from build123d import *

# Parameters (mm, degrees)
BASE_EXTRUDE_DEPTH = 10.5
FILLET1_R          = 1
SHELL1_START       = 43.20219293
SHELL1_OUTLINE_W   = 8
SHELL1_OUTLINE_H   = 19
SHELL1_DEPTH       = 9


# Read off the part's stored shape, not the designer's step: Shell1
with BuildPart() as part:
    # Sketch1 → Base-Extrude (new, symmetric)
    with BuildSketch(Plane.XY):
        Polygon((17.372143532, -52.78377934), (11.062802732, -43.773106853), (17.616019086, -39.184495362), (23.925359886, -48.195167849), align=None)
    extrude(amount=BASE_EXTRUDE_DEPTH, both=True)

    # Fillet1
    fillet1_edges = [part.edges().sort_by_distance(p)[0] for p in [
        (20.648751709, -50.489473594, 10.5),
        (20.770689486, -43.689831605, 10.5),
        (14.339410909, -41.478801107, 10.5),
        (20.770689486, -43.689831605, -10.5),
        (20.648751709, -50.489473594, -10.5),
        (14.217473132, -48.278443096, -10.5),
        (14.339410909, -41.478801107, -10.5),
        (14.217473132, -48.278443096, 10.5),
        (17.616019086, -39.184495362, 0),
        (23.925359886, -48.195167849, 0),
        (17.372143532, -52.78377934, 0),
        (11.062802732, -43.773106853, 0),
    ]]
    fillet(fillet1_edges, radius=FILLET1_R)

    # Shell1 outline → Shell1 (cut)
    with BuildSketch(Plane(origin=(0, 0, 0), x_dir=(0.8191520442889926, 0.5735764363510448, 0), z_dir=(0.5735764363510448, -0.8191520442889927, 0)).offset(SHELL1_START)):
        with Locations((-12.045105163, 0)):
            Rectangle(SHELL1_OUTLINE_W, SHELL1_OUTLINE_H)
    extrude(amount=SHELL1_DEPTH, mode=Mode.SUBTRACT)


solid = part.part
Verification items for the finished model (mm, model axes). A direction names the side the tool comes from. Round coordinates to 2 decimals unless told otherwise and drop trailing zeros. Loops run counter-clockwise (first coordinate to the right, second up) from the corner with the lowest first, then second, coordinate; pieces in that order, holes last. Notation, with made-up numbers: (17.5, 70) - (64.5, 70) arc R20 ccw to (64.5, 88) - close; hole circle Ø2 at (73.25, 53). An arc over 180 degrees is marked (long way). Write item = value, one per line.
Q1. Depth check by flat-ended pin: pin 1 (4 mm diameter, centred on y = -41, z = -0.5, fed in from -X); pin 2 (4 mm diameter, centred on x = 14.5, z = 3.5, fed in from +Y). Enter the tip coordinate at first touch or a pass-through.
Here are the results:
pin_1 = 12.17
pin_2 = -39.97
Q2. Material ranges on L1, parallel to Z at x = 20.5, y = -45; L2, parallel to Y at x = 17.25, z = 6.75; L3, parallel to Y at x = 17, z = 3.5, recorded low to high.
Here are the results:
L1 = -10.5 to -9.5, 9.5 to 10.5
L2 = -52.32 to -51.65, -40.66 to -39.58
L3 = -52.18 to -51.82, -40.84 to -39.65
Q3. Sectioned sample at A-A on z = -1.25. Record the boundary of the cut face in (x, y).
Here are the results:
outline = (11.64, -44.59) - (18.19, -40) arc R1 ccw to (16.8, -39.76) - (11.88, -43.2) arc R1 ccw to start; (16.8, -51.96) arc R1 ccw to (18.19, -52.21) - (23.11, -48.77) arc R1 ccw to (23.35, -47.38) - close
Q4. Tool access check on faces 1 (the cylindrical face through (20.56, -43.914, 10.215)), 2 (the flat face through (17, -46, 9.5)). Record the directions out of +Z, -Z, +X, -X, +Y, -Y that give a thin tool (end or side, any length) a straight path to the whole face; none if there is none.
Here are the results:
face_1 = +Z, +X, +Y
face_2 = none
Q5. Mould release check, pull along Z, two halves, no side actions. Record for faces 3 (the flat face through (17, -46, -9.5)), 4 (the flat face through (14.87, -42.33, 0.13)), 5 (the cylindrical face through (14.415, -48.063, -10.199)), 6 (the cylindrical face through (14.415, -48.063, 10.199)): +Z half, -Z half, draft (parallel to the pull), parting line (faces both ways), or undercut.
Here are the results:
face_3 = undercut
face_4 = undercut
face_5 = -Z half
face_6 = +Z half
